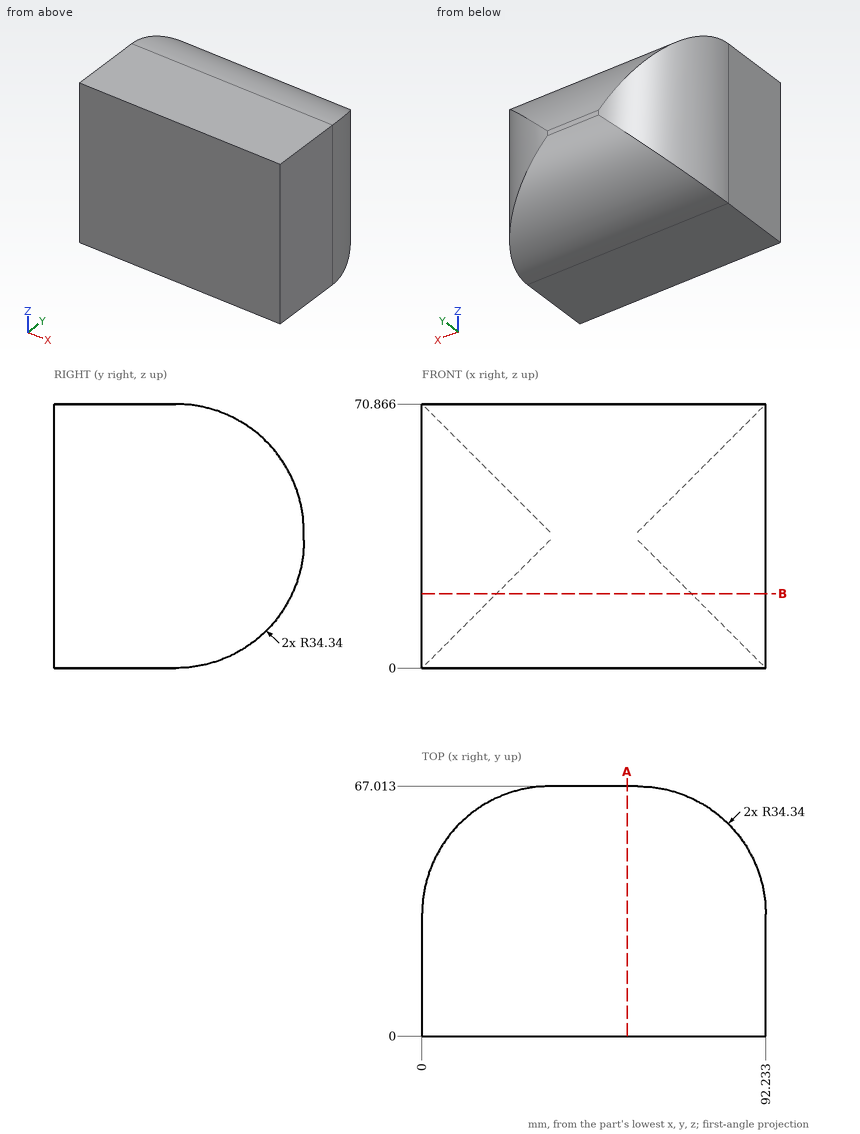
Drawing for the job (mm, zero at the part's lowest x, y, z). Give positions to 0.01 mm unless a question says otherwise; leave off trailing zeros. Order: outer loops, then holes, each group sorted by start corner. A loop starts at its lowest first (then second) coordinate and runs counter-clockwise, first axis right, second up. Notation, with made-up numbers: (-17, 4) - (38, 4) arc R24 ccw to (38, 39) - close; hole circle Ø1 at (43, 11.5). An arc over 180 degrees is marked (long way). Use one line per item in the form item = value.
Item 1: Probe probe 1 along Y at (x, z) = (29, 27); probe 2 along Y at (x, z) = (26, 30.5) (1 decimal); probe 3 along X at (y, z) = (38.5, 21.5) (1 decimal). List the from-to ranges inside material, lowest first. Write a range as from..to.
Solution:
probe_1 = 0..66.22
probe_2 = 0..66
probe_3 = 0.5..91.7
Item 2: Slice it at A-A on x = 55. Give the cut face in (y, z).
Solution:
outline = (0, 0) - (32.67, 0) arc R34.34 ccw to (67.01, 34.34) - (67.01, 36.53) arc R34.34 ccw to (32.67, 70.87) - (0, 70.87) - close
Item 3: Slice it at B-B on z = 20. Give the cut face in (x, y), and give its area (3 significant figures).
Solution:
outline = (0, 0) - (92.23, 0) - (92.23, 32.67) arc R34.34 ccw to (72.23, 63.88) - (20, 63.88) arc R34.34 ccw to (0, 32.67) - close
area = 5,540 mm2
Item 4: Pin check, flat tips, straight feed: pin 1 Ø1 at (x, z) = (58.5, 10.5) entering from +Y; pin 2 Ø10 at (x, y) = (76.5, 40.5) entering from -Z; pin 3 Ø12 at (y, z) = (48, 36.5) entering from +X. Stop position of each tip, or through.
Solution:
pin_1 = 57.86
pin_2 = 0.12
pin_3 = 90.94
